For this review, take the finished solid that the model builds, in its own axes (mm). Coordinates: 2 decimals unless noted, no trailing zeros. Loops run counter-clockwise (first coordinate to the right, second up) from the corner with the lowest first, then second, coordinate; pieces in that order, holes last. Notation, with made-up numbers: M 78.25,2 L 103.25,2 A18 ccw 103.25,10 Z; hole C 8,-0.5 d10. An arc over 180 degrees is marked long. Use one line per item in the form item = value.
Autodesk Inventor part; units mm, degrees
ref_plane "YZ Plane" through (0, 0, 0) normal (1, 0, 0) x (0, 1, 0)
ref_plane "XZ Plane" through (0, 0, 0) normal (0, 1, 0) x (-1, 0, 0)
ref_plane "XY Plane" through (0, 0, 0) normal (0, 0, 1) x (1, 0, 0)
sketch "Эскиз1" plane through (0, 0, 0) normal (0, 1, 0) x (-1, 0, 0)
  arc A0 (-0.25, 9.2247) -> (0.25, 9.2247) centre (0, 8) ccw
  line L0 (-0.25, 10.9972) -> (-0.25, 9.2247)
  arc A1 (-0.25, 10.9972) -> (-1.1469, -10.94) centre (0, 0) ccw
  line L1 (-1.1469, -10.6297) -> (-1.1469, -10.94)
  line L2 (-0.8473, -10.6297) -> (-1.1469, -10.6297)
  line L3 (-0.8473, -10.9673) -> (-0.8473, -10.6297)
  arc A2 (-0.8473, -10.9673) -> (0.8535, -10.9668) centre (0, 0) ccw
  line L4 (0.8535, -10.6297) -> (0.8535, -10.9668)
  line L5 (1.1541, -10.6297) -> (0.8535, -10.6297)
  line L6 (1.1541, -10.9393) -> (1.1541, -10.6297)
  arc A3 (1.1541, -10.9393) -> (0.25, 10.9972) centre (0, 0) ccw
  line L7 (0.25, 9.2247) -> (0.25, 10.9972)
  circle A4 centre (8, 0) radius 1.25
  circle A5 centre (0, -8) radius 1.25
  circle A6 centre (-8, 0) radius 1.25
  circle A7 centre (0, -5.5) radius 0.75
  circle A8 centre (4.7631, 2.75) radius 0.75
  circle A9 centre (-4.7631, 2.75) radius 0.75
  circle A10 centre (0, 0) radius 2.9
  arc A11 (0.25, 9.2247) -> (-0.25, 9.2247) centre (0, 8) ccw
  line L8 (0.25, 10.9972) -> (-0.25, 10.9972)
  line L9 (1.1541, -10.9393) -> (0.8535, -10.9668)
  line L10 (-0.8473, -10.9673) -> (-1.1541, -10.9393)
extrude "Выдавливание1" add sketch "Эскиз1" along normal blind 5 contours A0 L7 A3 L6 L5 L4 A2 L3 L2 L1 A1 L0 | L0 L8 L7 A11 | L9 L4 L5 L6 | L1 L2 L3 L10 | A7 | A8 | A9
sketch "Эскиз2" plane through (0, 5, 0) normal (0, 1, 0) x (1, 0, 0)
  circle A0 centre (0, -8) radius 1.25
  circle A1 centre (0, -8) radius 1.5
  circle A2 centre (-8, 0) radius 1.25
  circle A3 centre (-8, 0) radius 1.5
  circle A4 centre (0, 8) radius 1.25
  circle A5 centre (0, 8) radius 1.5
  circle A6 centre (8, 0) radius 1.25
  circle A7 centre (8, 0) radius 1.5
  point P0 (0, 0)
  dimension "d2" = 3
  dimension "d3" = 3
  dimension "d4" = 3
  dimension "d5" = 3
extrude "Выдавливание2" cut sketch "Эскиз2" against normal blind 10 contours A0 | A1 | A2 | A3 | A4 | A5 | A6 | A7
properties part number "проставка"
1. Consider section B-B on x = -8.5. Write out the cut boundary in (y, z), plus the area to 3 significant figures.
Computed values:
outline = M 0,-6.98 L 5,-6.98 L 5,-1.41 L 0,-1.41 Z; M 0,1.41 L 5,1.41 L 5,6.98 L 0,6.98 Z
area = 55.7 mm2
2. Consider section C-C on y = 0.85. Write out the cut boundary in (x, z), plus the area to 3 significant figures.
Computed values:
outline = M -1.15,-10.94 L -0.85,-10.97 A11 ccw 0.85,-10.97 L 1.15,-10.94 A11 ccw 0.25,11 L -0.25,11 A11 ccw Z; hole C -8,0 d3; hole C 0,0 d5.8; hole C 0,-8 d3; hole C 0,8 d3; hole C 8,0 d3
area = 325 mm2
3. For pin 1 Ø2.5 at (x, z) = (0, -8) entering from -Y; pin 2 Ø1 at (x, y) = (6, 3.5) entering from -Z, all flat-tipped, find the tip position at first contact; note any pin that passes through.
Computed values:
pin_1 = through
pin_2 = -9.53
4. Consider section A-A on z = 0.5. Write out the cut boundary in (x, y).
Computed values:
outline = M -10.99,0 L -9.41,0 L -9.41,5 L -10.99,5 Z; M -6.59,0 L -2.86,0 L -2.86,5 L -6.59,5 Z; M 2.86,0 L 6.59,0 L 6.59,5 L 2.86,5 Z; M 9.41,0 L 10.99,0 L 10.99,5 L 9.41,5 Z
5. Draft analysis for pull direction Z (two halves, no side actions). For faces 1 (the face through (0, 2, -11)), 2 (the face through (-0.325, 2.535, -6.536)), 3 (the face through (-2.3, 5, -2.3)), state which applies: +Z half, -Z half, draft (parallel to the pull), parting line (faces both ways), or undercut.
Computed values:
face_1 = -Z half
face_2 = undercut
face_3 = draft
6. Consider section D-D on z = 7.5. Write out the cut boundary in (x, y), plus the area to 3 significant figures.
Computed values:
outline = M -8.05,0 L -1.41,0 L -1.41,5 L -8.05,5 Z; M 1.41,0 L 8.05,0 L 8.05,5 L 1.41,5 Z
area = 66.3 mm2
7. Wall thickness on line 1 along Z through (x, y) = (0, 3.2); line 2 along X through (y, z) = (4.7, 7); line 3 along Z through (x, y) = (8, 1.5): over which ranges is each line inside the solid? List them lowest first. Write a range as from..to.
Computed values:
line_1 = -11..-9.5, -6.5..-2.9, 2.9..6.5, 9.5..11
line_2 = -8.49..-1.12, 1.12..8.49
line_3 = -7.55..-1.5, 1.5..7.55
